Autodesk Inventor part; units mm, degrees
ref_plane "Work Plane1" through (111.7581, 40.3852, 111.4201) normal (-0.9659258, 0.258819, 0) x (-0.1358803, -0.507112, -0.8511016)
ref_plane "YZ Plane" through (0, 0, 0) normal (1, 0, 0) x (0, 1, 0)
ref_plane "XZ Plane" through (0, 0, 0) normal (0, 1, 0) x (-1, 0, 0)
ref_plane "Work Plane1" through (111.7581, 40.3852, 111.4201) normal (-0.9659258, 0.258819, 0) x (-0.1358803, -0.507112, -0.8511016)
sketch "Sketch1" plane through (111.7581, 40.3852, 111.4201) normal (-0.9659258, 0.258819, 0) x (-0.1358803, -0.507112, -0.8511016)
  line L0 (0, -6.3437) -> (253.9995, -6.3437) construction
  line L1 (228.4809, -42.564) -> (250.8233, -6.3437) construction
  line L2 (108.9501, -41.6524) -> (130.3466, -6.9656) construction
  line L3 (107.0353, -38.7089) -> (126.9998, -6.3437) construction
  line L4 (-20.5605, -41.6524) -> (-3.3186, -13.7009) construction
  line L5 (-4.9348, -10.2733) -> (-23.2434, -39.9543) construction
  line L6 (-3.3186, -13.7009) -> (1.2196, -6.3437) construction
  line L7 (130.3466, -6.9656) -> (130.7302, -6.3437) construction
  line L8 (130.7302, -6.3437) -> (250.8233, -6.3437)
  line L9 (126.9998, -6.3437) -> (1.2196, -6.3437)
  line L10 (-20.5605, -41.6524) -> (108.9501, -41.6524) construction
  line L11 (108.9501, -41.6524) -> (232.7736, -41.6524) construction
  line L12 (107.0353, -38.7089) -> (105.2196, -41.6524) construction
  line L13 (229.0432, -41.6524) -> (250.8233, -6.3437)
  line L14 (229.0432, -41.6524) -> (108.9501, -41.6524)
  line L15 (130.7302, -6.3437) -> (108.9501, -41.6524)
  line L16 (105.2196, -41.6524) -> (126.9998, -6.3437)
  line L17 (105.2196, -41.6524) -> (-20.5605, -41.6524)
  line L18 (-20.5605, -41.6524) -> (1.2196, -6.3437)
  line L19 (120.3322, -17.1527) -> (123.0345, -18.8196)
  line L20 (113.6647, -27.9617) -> (116.367, -29.6286)
  line L21 (244.1558, -17.1527) -> (246.8581, -18.8196)
  line L22 (246.8581, -18.8196) -> (240.1905, -29.6286)
  line L23 (240.1905, -29.6286) -> (237.4883, -27.9617)
  line L24 (-5.4479, -17.1527) -> (-8.1501, -15.4858)
  line L25 (-8.1501, -15.4858) -> (-14.8176, -26.2948)
  line L26 (-14.8176, -26.2948) -> (-12.1154, -27.9617)
  line L27 (256.5554, -3.0988) -> (232.2107, -42.5651) construction
  line L28 (105.2196, -41.6524) -> (134.1991, 5.3274) construction
  line L29 (136.9013, 3.6606) -> (107.9219, -43.3193) construction
  line L30 (12.8127, 12.4503) -> (-20.8503, -42.1222) construction
  line L31 (-23.5525, -40.4553) -> (10.1104, 14.1172) construction
  line L32 (256.5554, -3.0988) -> (232.2107, -42.5651) construction
  line L33 (237.4883, -27.9617) -> (229.5084, -40.8982) construction
  line L34 (250.8233, -6.3437) -> (244.1558, -17.1527) construction
  point P0 (126.9998, -6.3437)
  dimension "d0" = 12.7
  dimension "d1" = 12.7
  dimension "d2" = 12.7
  dimension "d3" = 12.7
  dimension "d4" = 12.7
  dimension "d5" = 12.7
extrude "Extrusion1" add sketch "Sketch1" along normal blind 3.175
sketch "Sketch2" plane through (111.7581, 40.3852, 111.4201) normal (0.9659258, -0.258819, 0) x (-0.1358803, -0.507112, -0.8511016)
  line L0 (-20.5605, 41.6524) -> (105.2196, 41.6524) construction
  line L1 (42.3296, 41.6524) -> (64.1097, 6.3437) construction
  line L2 (126.9998, 6.3437) -> (1.2196, 6.3437) construction
  line L3 (108.9501, 41.6524) -> (229.0432, 41.6524) construction
  line L4 (168.9966, 41.6524) -> (190.7768, 6.3437) construction
  line L5 (250.8233, 6.3437) -> (130.7302, 6.3437) construction
  point P0 (130.4954, 0.6768)
  point P1 (53.2196, 23.9981)
  point P2 (179.8867, 23.9981)
hole "Hole1" at (109.8129, 33.1257, 53.5258) at (92.6013, -31.1087, -54.2807) direction (-0.9659258, 0.258819, 0) diameter 6.7564 depth 13.6144
sketch "Sketch3" plane through (111.7581, 40.3852, 111.4201) normal (0.9659258, -0.258819, 0) x (-0.1358803, -0.507112, -0.8511016)
  line L0 (-8.1501, 15.4858) -> (-14.8176, 26.2948)
  line L1 (-11.4839, 20.8903) -> (6.8914, 32.2251) construction
  line L2 (5.2245, 34.9273) -> (-13.1507, 23.5925)
  line L3 (-8.1501, 15.4858) -> (-14.8176, 26.2948)
  line L4 (-9.817, 18.1881) -> (8.5583, 29.5228)
  line L5 (2.7826, 23.1623) -> (-3.0515, 32.6201)
  line L6 (-3.0515, 32.6201) -> (-7.3751, 29.9531)
  line L7 (-7.3751, 29.9531) -> (-1.541, 20.4953)
  line L8 (-1.541, 20.4953) -> (2.7826, 23.1623)
  line L9 (-7.3751, 29.9531) -> (2.7826, 23.1623) construction
  line L10 (240.1905, 29.6286) -> (246.8581, 18.8196)
  line L11 (243.5243, 24.2241) -> (225.149, 12.8893) construction
  line L12 (5.2245, 34.9273) -> (8.5583, 29.5228)
  line L13 (223.4821, 15.5915) -> (226.8159, 10.187)
  line L14 (226.8159, 10.187) -> (245.1912, 21.5218)
  line L15 (223.4821, 15.5915) -> (241.8574, 26.9263)
  line L16 (239.4155, 15.1612) -> (235.0919, 12.4942)
  line L17 (235.0919, 12.4942) -> (229.2578, 21.9521)
  line L18 (229.2578, 21.9521) -> (233.5814, 24.6191)
  line L19 (233.5814, 24.6191) -> (239.4155, 15.1612)
  line L20 (239.4155, 15.1612) -> (229.2578, 21.9521) construction
  line L21 (-14.4934, 26.4948) -> (-7.8258, 15.6858)
  line L22 (-14.8176, 26.2948) -> (-12.1154, 27.9617)
  line L23 (-5.4479, 17.1527) -> (-8.1501, 15.4858)
  line L24 (239.8663, 29.4285) -> (246.584, 18.5381)
  line L25 (246.8581, 18.8196) -> (244.1558, 17.1527)
  line L26 (237.4883, 27.9617) -> (240.1905, 29.6286)
  point P0 (130.4954, 0.6768)
  point P1 (-2.2962, 26.5577)
  point P2 (234.3367, 18.5567)
  point P3 (1.5325, 25.1889)
  point P4 (-1.8013, 30.5934)
  point P5 (-6.1249, 27.9264)
  point P6 (-9.817, 18.1881)
  point P7 (-2.7911, 22.5219)
  point P8 (238.1653, 17.1879)
  point P9 (234.8316, 22.5924)
  point P10 (230.508, 19.9254)
  point P11 (233.8417, 14.5209)
  point P12 (241.5332, 26.7263)
  point P13 (246.5338, 18.6195)
  point P14 (244.8669, 21.3218)
  point P15 (-12.8265, 23.7926)
  point P16 (-9.4927, 18.3881)
  dimension "d16" = 21.59
  dimension "d19" = 11.1125
  dimension "d20" = 5.08
  dimension "d21" = 21.59
  dimension "d22" = 6.35
  dimension "d23" = 6.35
  dimension "d24" = 5.08
  dimension "d25" = 11.1125
  dimension "d28" = 0.381
  dimension "d29" = 0.381
extrude "Extrusion2" cut sketch "Sketch3" against normal through all
properties part number "SidePlate" material "Aluminum 6061"
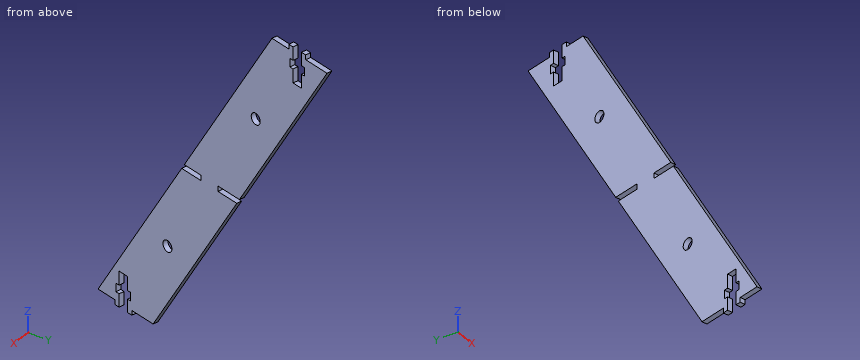
Build history of the part. All positions in model axes, mm. Round coordinates to 2 decimals unless told otherwise and drop trailing zeros. Write each loop counter-clockwise with the first axis right and the second up, starting at its lowest first coordinate (ties: lowest second). Pieces come first, ordered by that corner, then holes. Notation, with made-up numbers: M 26.5,16 L 31.5,16 A20 cw 31.5,50 Z; hole C 64,-10 d6. An arc over 180 degrees is marked long. Answer as a JSON object with one key per item and string values. Group by question number.
(1) Cut at B-B (y = 75). Give the cut face in (x, z), and give its area (3 significant figures).
(2) Cut at C-C (z = -79.5). Give the cut face in (x, y).
(3) Drill centre lines: L1, parallel to Z at x = 115.5, y = 60; L2, parallel to X at y = 34.5, z = 62.5; L3, parallel to X at y = 26, z = 14. Where is each one in solid material? Low to high.
(4) Cut at A-A (z = -55). Give the cut face in (x, y).
(5) Flat gauge pins, fed straight in: pin 1 (0.9 mm diameter, centred on x = 117, y = 68.5, fed in from -Z); pin 2 (8 mm diameter, centred on x = 120.5, y = 76, fed in from +Z); pin 3 (7 mm diameter, centred on x = 95, y = -12, fed in from -Z). Where does each tip first touch, or does it go through?
Responses:
{
 "1": {"outline": "M 117.75,88.8 L 121.03,90.18 L 121.03,107.05 L 117.75,107.05 Z", "area": "57.7 mm2"},
 "2": {"outline": "M 80.14,-65.35 L 83.21,-66.17 L 93.94,-26.1 L 90.88,-25.28 Z"},
 "3": {"L1": "z = 64.37 to 96.89, 101.97 to 109.85", "L2": "x = 106.89 to 110.18", "L3": "x = 104.62 to 107.9"},
 "4": {"outline": "M 84.05,-50.75 L 87.12,-51.57 L 91.75,-34.3 L 88.68,-33.48 Z; M 90.39,-27.1 L 93.46,-27.92 L 97.86,-11.5 L 94.79,-10.68 Z"},
 "5": {"pin 1": "stops at z = 77.58", "pin 2": "stops at z = 107.05", "pin 3": "stops at z = -62.65"}
}
